from build123d import *

# Parameters (mm, degrees)
SKETCH_R  = 1
PAD_DEPTH = 2


with BuildPart() as part:
    # Sketch → Pad (new body)
    with BuildSketch(Plane.XY):
        with BuildLine():
            ThreePointArc((0, 50), (-25, 25), (0, 0))
            Line((2, 0), (0, 0))
            Line((2, -20.5), (2, 0))
            ThreePointArc((2, -20.5), (0.5, -22), (2, -23.5))
            Line((2, -23.5), (2, -24.5))
            Line((2, -24.5), (-2, -24.5))
            Line((-2, -4), (-2, -24.5))
            ThreePointArc((0, 51.5), (-27.768012, 24.714613), (-2, -4))
            Line((0, 50), (0, 51.5))
        make_face()
        with Locations((0, -2)):
            Circle(SKETCH_R, mode=Mode.SUBTRACT)
    extrude(amount=PAD_DEPTH)


solid = part.part
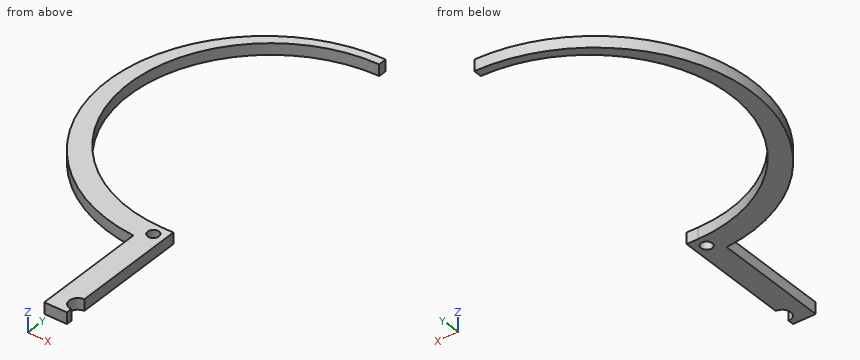
The listing builds one solid part. Answer for the finished solid, in the listing's coordinates (mm). Give positions to 0.01 mm unless a question says otherwise; leave off trailing zeros. Loops run counter-clockwise (first coordinate to the right, second up) from the corner with the lowest first, then second, coordinate; pieces in that order, holes last. Notation, with made-up numbers: (87, 0) - (96, 0) arc R10 cw to (96, 6) - close; hole circle Ø1 at (12.25, -36). An arc over 180 degrees is marked (long way). Write each question's results on one line, items separated by ' | '.
1. Find section B-B, the plane y = -2. Write down the section's boundary in (x, z), then the cut area to 3 significant figures.
Resolved:
outline: (-10.53, 0) - (-1, 0) - (-1, 2) - (-10.53, 2) - close; (1, 0) - (2, 0) - (2, 2) - (1, 2) - close | area: 21.1 mm^2
2. Consider probe 1 along Y at (x, z) = (-15.25, 1.7); probe 2 along Y at (x, z) = (-14.5, 0.5); probe 3 along X at (y, z) = (22.5, 1.35). Determine where each line is inside the solid, lowest interval first. Write a range as from..to.
Resolved:
probe 1: y = 0.49..5.19, 44.81..46.94 | probe 2: y = 0.01..4.63, 45.37..47.42 | probe 3: x = -27.76..-24.87
3. Flat-ended cylindrical pins translate along their axes: P1, Ø0.6, axis at x = 1, z = 1.5, coming from the +Y side; P2, Ø1, axis at y = -18.5, z = 1, coming from the -X side; P3, Ø1.2, axis at y = 50.5, z = 1.5, coming from the +X side. Find the tip coordinate at first contact, or state that the pin passes through.
Resolved:
P1: stops at y = 0 | P2: stops at x = -2 | P3: stops at x = 0
4. Find section D-D, the plane y = -10. Write down the section's boundary in (x, z), then the cut area to 3 significant figures.
Resolved:
outline: (-2, 0) - (2, 0) - (2, 2) - (-2, 2) - close | area: 8.00 mm^2
5. Find section C-C, the plane x = -18.5. Write down the section's boundary in (y, z).
Resolved:
outline: (2.98, 0) - (8.18, 0) - (8.18, 2) - (2.98, 2) - close; (41.82, 0) - (44.45, 0) - (44.45, 2) - (41.82, 2) - close
